from build123d import *

# Parameters (mm, degrees)
SKETCH1_W            = 200
SKETCH1_H            = 150
BOSS_EXTRUDE1_DEPTH  = 300
SKETCH2_R            = 10
BOSS_EXTRUDE2_DEPTH  = 10
LPATTERN1_COUNT      = 2
LPATTERN1_PITCH      = 135
LPATTERN1_COUNT_DIR2 = 2
LPATTERN1_PITCH_DIR2 = 95
SKETCH3_W            = 60
SKETCH3_H            = 85
BOSS_EXTRUDE3_DEPTH  = 2
SKETCH4_R            = 6.5
SKETCH4_R_2          = 4.5
SKETCH4_R_3          = 5.5
CUT_EXTRUDE1_DEPTH   = 10
SKETCH5_W            = 40
SKETCH5_H            = 30
BOSS_EXTRUDE4_DEPTH  = 2
SKETCH6_W            = 12
SKETCH6_H            = 7
CUT_EXTRUDE2_DEPTH   = 10
LPATTERN2_COUNT      = 2
LPATTERN2_PITCH      = 20
LPATTERN2_COUNT_DIR2 = 2
LPATTERN2_PITCH_DIR2 = 15
SWEEP1_PROFILE_R     = 15
SWEEP3_PROFILE_R     = 15


with BuildPart() as part:
    # Sketch1 → Boss-Extrude1 (new body)
    with BuildSketch(Plane(origin=(0, 0, 0), x_dir=(1, 0, 0), z_dir=(0, 1, 0))):
        with Locations((100, 75)):
            Rectangle(SKETCH1_W, SKETCH1_H)
    extrude(amount=BOSS_EXTRUDE1_DEPTH)

    # Sketch2 → Boss-Extrude2 (add)
    with BuildSketch(Plane.XZ):
        with Locations(Location((30, -30, 0), (0, 0, 270))):
            Circle(SKETCH2_R)
    boss_extrude2 = extrude(amount=BOSS_EXTRUDE2_DEPTH)

    # LPattern1: Boss-Extrude2 2 × 2
    with Locations(*[(i * LPATTERN1_PITCH, 0, -j * LPATTERN1_PITCH_DIR2) for i in range(LPATTERN1_COUNT) for j in range(LPATTERN1_COUNT_DIR2) if (i, j) != (0, 0)]):
        add(boss_extrude2)

    # Sketch3 → Boss-Extrude3 (add)
    with BuildSketch(Plane(origin=(200, 0, 0), x_dir=(0, 0, -1), z_dir=(1, 0, 0))):
        with Locations((73, 156.159254336)):
            Rectangle(SKETCH3_W, SKETCH3_H)
    extrude(amount=BOSS_EXTRUDE3_DEPTH)

    # Sketch4 → Cut-Extrude1 (cut)
    with BuildSketch(Plane(origin=(202, 0, 0), x_dir=(0, 0, -1), z_dir=(1, 0, 0))):
        with Locations((71.853020993, 175.943431477)):
            Circle(SKETCH4_R)
        with Locations((57.356733942, 154.567450344)):
            Circle(SKETCH4_R_2)
        with Locations((87.212182272, 154.567450344)):
            Circle(SKETCH4_R_2)
        with Locations((52.869787951, 137.459240855)):
            Circle(SKETCH4_R_3)
        with Locations((91.353978572, 137.459240855)):
            Circle(SKETCH4_R_3)
    extrude(amount=-CUT_EXTRUDE1_DEPTH, mode=Mode.SUBTRACT)

    # Sketch5 → Boss-Extrude4 (add)
    with BuildSketch(Plane(origin=(200, 0, 0), x_dir=(0, 0, -1), z_dir=(1, 0, 0))):
        with Locations((45.757145197, 234.416332146)):
            Rectangle(SKETCH5_W, SKETCH5_H)
    extrude(amount=BOSS_EXTRUDE4_DEPTH)

    # Sketch6 → Cut-Extrude2 (cut)
    with BuildSketch(Plane(origin=(202, 0, 0), x_dir=(0, 0, -1), z_dir=(1, 0, 0))):
        with Locations((35.621192249, 242.789266553)):
            Rectangle(SKETCH6_W, SKETCH6_H)
    cut_extrude2 = extrude(amount=-CUT_EXTRUDE2_DEPTH, mode=Mode.SUBTRACT)

    # LPattern2: Cut-Extrude2 2 × 2
    with Locations(*[(0, -j * LPATTERN2_PITCH_DIR2, -i * LPATTERN2_PITCH) for i in range(LPATTERN2_COUNT) for j in range(LPATTERN2_COUNT_DIR2) if (i, j) != (0, 0)]):
        add(cut_extrude2, mode=Mode.SUBTRACT)

    # Sweep1: sweep along a curve in space
    with BuildLine() as sweep1_path:
        Line((44.183408536, 300, -78.446799091), (44.183408536, 339.05786042, -78.446799091))
        ThreePointArc((44.183408536, 339.05786042, -78.446799091), (52.970205101, 360.271063856, -78.446799091), (74.183408536, 369.05786042, -78.446799091))
        Line((74.183408536, 369.05786042, -78.446799091), (118.129151449, 369.05786042, -78.446799091))
        ThreePointArc((118.129151449, 369.05786042, -78.446799091), (139.550389075, 360.060969204, -78.446799091), (148.123323724, 338.466565659, -78.446799091))
        Line((148.123323724, 338.466565659, -78.446799091), (147.365007124, 300, -78.446799091))
    # Sweep1 profile (on start of the path) → Sweep1 (sweep)
    with BuildSketch(Plane(origin=(44.183408536, 300, -78.446799091), x_dir=(0, 0, 1), z_dir=(0, 1, 0))):
        Circle(SWEEP1_PROFILE_R)
    sweep(path=sweep1_path.line)

    # Sweep3: sweep along a curve in space
    with BuildLine() as sweep3_path:
        Line((0, 196.29190753, -76.403481412), (-68.808571034, 196.29190753, -76.403481412))
        ThreePointArc((-68.808571034, 196.29190753, -76.403481412), (-79.81229202, 191.489875152, -76.208825939), (-83.764863748, 180.160905025, -75.749594126))
        Line((-83.764863748, 180.160905025, -75.749594126), (-74.792635523, 62.982710481, -70.999651793))
        ThreePointArc((-74.792635523, 62.982710481, -70.999651793), (-78.745207251, 51.653740354, -70.540419979), (-89.748928238, 46.851707976, -70.345764506))
        Line((-89.748928238, 46.851707976, -70.345764506), (-173.557499271, 46.851707976, -70.345764506))
    # Sweep3 profile (on start of the path) → Sweep3 (sweep)
    with BuildSketch(Plane(origin=(0, 196.29190753, -76.403481412), x_dir=(0, 0, -1), z_dir=(-1, 0, 0))):
        Circle(SWEEP3_PROFILE_R)
    sweep(path=sweep3_path.line)


solid = part.part
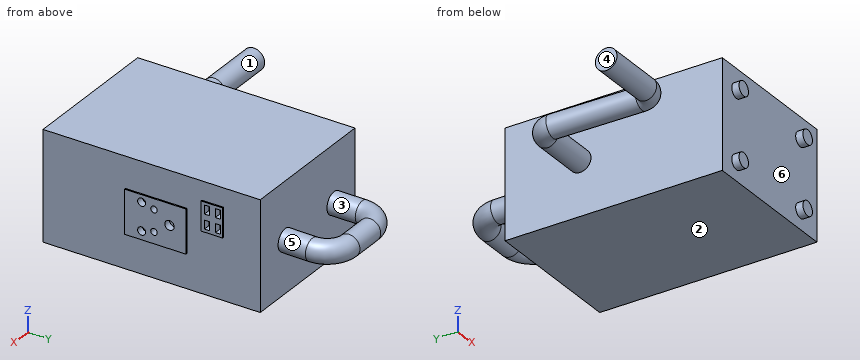
Model file for the job. Use its own axes, mm. Face numbers are marked on the shaded views. A direction names the side the tool comes from. Give positions to 0.01 mm unless a question says otherwise; leave off trailing zeros. Write each loop counter-clockwise with the first axis right and the second up, starting at its lowest first coordinate (ties: lowest second). Pieces come first, ordered by that corner, then holes. Notation, with made-up numbers: (60.5, 59) - (113.5, 59) arc R35 cw to (113.5, 94) - close; hole circle Ø6 at (27.25, -3). An arc over 180 degrees is marked (long way). Answer as CSV lines item,"result".
1. Two-plate mould, pull along Y, no slides. Class the marked faces 4, 5 and 6: +Y half, -Y half, draft (parallel to the pull), parting line (faces both ways), or undercut.
Responses:
face 4,"draft"
face 5,"undercut"
face 6,"-Y half"
2. Band-saw the part on A-A (z = -125). Write the cut outline in (x, y).
Responses:
outline,"(0, 0) - (20, 0) - (20, -10) - (40, -10) - (40, 0) - (155, 0) - (155, -10) - (175, -10) - (175, 0) - (200, 0) - (200, 300) - (0, 300) - close"
3. 3-axis set-ups, long thin cutter, end or side, ignore diameter. For the marked faces 1, 2 and 3: which of +Z, -Z, +X, -X, +Y, -Y reach the whole face in a straight line?
Responses:
face 1,"-X"
face 2,"-Z, +X, -X, +Y, -Y"
face 3,"none"
4. Pin check, flat tips, straight feed: pin 1 (6 mm diameter, centred on x = 119, z = -132.5, fed in from +Y); pin 2 (5 mm diameter, centred on x = -58.5, y = 210, fed in from -Z); pin 3 (10.5 mm diameter, centred on y = 175.94, z = -71.85, fed in from +X). Stop position of each tip, or through.
Responses:
pin 1,"stops at y = 300"
pin 2,"stops at z = -86.37"
pin 3,"stops at x = 192"
5. Band-saw the part on B-B (y = 263). Write the cut outline in (x, z), and give its area (3 significant figures).
Responses:
outline,"(0, -150) - (200, -150) - (200, 0) - (0, 0) - close"
area,"30,000 mm2"
6. Drill centre lines: L1, parallel to X at y = 90, z = -128; L2, parallel to Y at x = 8, z = -102.5; L3, parallel to X at y = 230.5, z = -26. Where is each one in solid material? Low to high. Write a range as [from, to].
Responses:
L1,"x = [0, 200]"
L2,"y = [0, 300]"
L3,"x = [0, 202]"
7. Band-saw the part on C-C (x = -118). Write the cut outline in (y, z).
Responses:
outline,"circle Ø30 at (46.85, -70.35)"
